```python
from build123d import *

# Parameters (mm, degrees)
EXTRUDE_THIN1_DEPTH = 12.2
SKETCH2_R           = 1.3
CUT_EXTRUDE1_DEPTH  = 28.957288853
SKETCH3_W           = 2
SKETCH3_H           = 10
BOSS_EXTRUDE1_DEPTH = 12.2
FILLET1_R           = 2
SKETCH4_R           = 1.5
CUT_EXTRUDE2_DEPTH  = 32.186695881
SKETCH5_W           = 12.2
SKETCH5_H           = 2
BOSS_EXTRUDE2_DEPTH = 5
SKETCH8_R           = 1.6
CUT_EXTRUDE4_DEPTH  = 3
BOSS_EXTRUDE3_START = 11.4
SKETCH9_W           = 12.2
SKETCH9_H           = 4
SKETCH9_R           = 1.5
BOSS_EXTRUDE3_DEPTH = 11.4
SKETCH10_R          = 1.5
SKETCH10_R_2        = 1.6
CUT_EXTRUDE5_DEPTH  = 12
SKETCH12_R          = 1.9
BOSS_EXTRUDE5_DEPTH = 8
SKETCH13_W          = 1
SKETCH13_H          = 4
CUT_EXTRUDE6_DEPTH  = 37.592485601
FILLET4_R           = 0.5
CUT_EXTRUDE7_REACH  = 38.592
SKETCH14_W          = 4.5
SKETCH14_H          = 1.8
CUT_EXTRUDE8_REACH  = 47.951
SKETCH15_W          = 6
SKETCH15_H          = 8.2


with BuildPart() as part:
    # Sketch1 → Extrude-Thin1 (new body)
    with BuildSketch(Plane(origin=(0, 0, 0), x_dir=(0, 0, -1), z_dir=(1, 0, 0))):
        Polygon((0, 16.6), (0, 11.6), (-18.9, 11.6), (-18.9, -11.6), (0, -11.6), (0, -16.6), (-2, -16.6), (-2, -13.6), (-20.9, -13.6), (-20.9, 13.6), (-2, 13.6), (-2, 16.6), align=None)
    extrude(amount=EXTRUDE_THIN1_DEPTH)

    # Sketch2 → Cut-Extrude1 (cut, through all)
    with BuildSketch(Plane(origin=(0, 0, 18.9), x_dir=(-1, 0, 0), z_dir=(0, 0, -1))):
        with Locations(Location((-6.05, -5.15, 0), (0, 0, 90))):
            Circle(SKETCH2_R)
    extrude(amount=-CUT_EXTRUDE1_DEPTH, mode=Mode.SUBTRACT)

    # Sketch3 → Boss-Extrude1 (add)
    with BuildSketch(Plane(origin=(12.2, 0, 0), x_dir=(0, 0, -1), z_dir=(1, 0, 0))):
        with Locations((-19.9, 16.6)):
            Rectangle(SKETCH3_W, SKETCH3_H)
    extrude(amount=-BOSS_EXTRUDE1_DEPTH)

    # Fillet1
    fillet1_edges = [part.edges().sort_by_distance(p)[0] for p in [
        (6.1, -13.6, 2),
        (6.1, 13.6, 2),
        (6.1, 13.6, 18.9),
    ]]
    fillet(fillet1_edges, radius=FILLET1_R)

    # Sketch4 → Cut-Extrude2 (cut, through all)
    with BuildSketch(Plane(origin=(0, 0, 18.9), x_dir=(-1, 0, 0), z_dir=(0, 0, -1))):
        with Locations((-6.1, 19.6)):
            Circle(SKETCH4_R)
    extrude(amount=-CUT_EXTRUDE2_DEPTH, mode=Mode.SUBTRACT)

    # Sketch5 → Boss-Extrude2 (add)
    with BuildSketch(Plane(origin=(0, 16.6, 0), x_dir=(1, 0, 0), z_dir=(0, 1, 0))):
        with Locations((6.1, -1)):
            Rectangle(SKETCH5_W, SKETCH5_H)
    extrude(amount=BOSS_EXTRUDE2_DEPTH)

    # Sketch8 → Cut-Extrude4 (cut)
    with BuildSketch(Plane.XY.offset(2)):
        with Locations((6.1, 19.6)):
            Circle(SKETCH8_R)
    extrude(amount=-CUT_EXTRUDE4_DEPTH, mode=Mode.SUBTRACT)

    # Sketch9 → Boss-Extrude3 (add)
    with BuildSketch(Plane(origin=(0, 0, 0), x_dir=(-1, 0, 0), z_dir=(0, 0, -1)).offset(BOSS_EXTRUDE3_START)):
        with Locations((-6.1, 19.6)):
            Rectangle(SKETCH9_W, SKETCH9_H)
        with Locations((-6.1, 19.6)):
            Circle(SKETCH9_R, mode=Mode.SUBTRACT)
    extrude(amount=-BOSS_EXTRUDE3_DEPTH)

    # Sketch10 → Cut-Extrude5 (cut)
    with BuildSketch(Plane(origin=(0, 0, 0), x_dir=(-1, 0, 0), z_dir=(0, 0, -1))):
        with Locations(Location((-6.05, -13.9, 0), (0, 0, 90))):
            Circle(SKETCH10_R)
        with Locations(Location((-6.05, 14.1, 0), (0, 0, 90))):
            Circle(SKETCH10_R_2)
    extrude(amount=-CUT_EXTRUDE5_DEPTH, mode=Mode.SUBTRACT)

    # Sketch12 → Boss-Extrude5 (add)
    with BuildSketch(Plane(origin=(0, 0, 18.9), x_dir=(-1, 0, 0), z_dir=(0, 0, -1))):
        with Locations(Location((-6.05, -5.35, 0), (0, 0, 90))):
            Circle(SKETCH12_R)
    extrude(amount=-BOSS_EXTRUDE5_DEPTH)

    # Sketch13 → Cut-Extrude6 (cut, through all)
    with BuildSketch(Plane(origin=(12.2, 0, 0), x_dir=(0, 0, -1), z_dir=(1, 0, 0))):
        with Locations((10.9, 19.6)):
            Rectangle(SKETCH13_W, SKETCH13_H)
    extrude(amount=-CUT_EXTRUDE6_DEPTH, mode=Mode.SUBTRACT)

    # Fillet4
    fillet4_edges = [part.edges().sort_by_distance(p)[0] for p in [
        (6.05, -7.25, 20.9),
    ]]
    fillet(fillet4_edges, radius=FILLET4_R)

    # Cut-Extrude7: up to this face of the body (flat: up to its plane)
    cut_extrude7_end = Plane(part.part.faces().sort_by_distance((6.1, 0, 18.9))[0])
    # Sketch14 → Cut-Extrude7 (cut, up to the picked face)
    with BuildSketch(Plane(origin=(0, 0, 0), x_dir=(-1, 0, 0), z_dir=(0, 0, -1)), mode=Mode.PRIVATE) as cut_extrude7_sk1:
        with Locations((-6.1, -12.5)):
            Rectangle(SKETCH14_W, SKETCH14_H)
    cut_extrude7_tool1 = split(extrude(cut_extrude7_sk1.sketch, amount=-CUT_EXTRUDE7_REACH, mode=Mode.PRIVATE), bisect_by=cut_extrude7_end, keep=Keep.BOTH, mode=Mode.PRIVATE)
    add(cut_extrude7_tool1.solids().sort_by(Axis((6.1, -12.5, 0), (0, 0, 1)))[0], mode=Mode.SUBTRACT)

    # Cut-Extrude8: up to this face of the body (flat: up to its plane)
    cut_extrude8_end = Plane(part.part.faces().sort_by_distance((1.925, -11.6, 9.45))[0])
    # Sketch15 → Cut-Extrude8 (cut, up to the picked face)
    with BuildSketch(Plane.XZ.offset(13.6), mode=Mode.PRIVATE) as cut_extrude8_sk1:
        with Locations((6.1, 14.3)):
            Rectangle(SKETCH15_W, SKETCH15_H)
    cut_extrude8_tool1 = split(extrude(cut_extrude8_sk1.sketch, amount=-CUT_EXTRUDE8_REACH, mode=Mode.PRIVATE), bisect_by=cut_extrude8_end, keep=Keep.BOTH, mode=Mode.PRIVATE)
    add(cut_extrude8_tool1.solids().sort_by(Axis((6.1, -13.6, 14.3), (0, 1, 0)))[0], mode=Mode.SUBTRACT)


solid = part.part
```
Build history of the part. All positions in model axes, mm. A direction names the side the tool comes from. Round coordinates to 2 decimals unless told otherwise and drop trailing zeros. Loops run counter-clockwise (first coordinate to the right, second up) from the corner with the lowest first, then second, coordinate; pieces in that order, holes last.
Item 1: Drill centre lines: line 1 along Y through (x, z) = (6.1, 0.85); line 2 along X through (y, z) = (-13.5, 16); line 3 along Z through (x, y) = (8.5, 17). Where is each one in solid material? Low to high.
Item 2: Which spindle directions (+Z, -Z, +X, -X, +Y, -Y) get a long thin tool onto all of the face, cutting with end or side? Do faces 5 (the face through (6, 11.6, 9)), 6 (the face through (8.35, -13, 5)), 7 (the face through (2.17, 14.2, 2.57)), 8 (the face through (6, 17.6, -5)). Say none if no direction does.
Item 3: Saw through at C-C (z = -6.5). List the corners of the cut face in (x, y).
Item 4: Saw through at D-D (y = -5.35). List the corners of the cut face in (x, z).
Item 5: Saw through at B-B (x = 1.75). List the corners of the cut face in (y, z), then the cut area to 3 significant figures.
Item 6: Pin check, flat tips, straight feed: P1, Ø0.5, axis at y = -12.5, z = 4, coming from the -X side; P2, Ø0.9, axis at x = 6.5, y = 13.5, coming from the -Z side; P3, Ø6, axis at x = 6, y = 9.5, coming from the +Z side; P4, Ø1, axis at x = 10, y = -10, coming from the -Z side. Stop position of each tip, or through.
Item 7: Two-plate mould, pull along Z, no slides. Class faces 1 (the face through (6.2, 17.9, 18.9)), 2 (the face through (6, 16, 0)), 3 (the face through (6, 21.6, -4)), 4 (the face through (6.01, 14.17, 18.3)): released by +Z, released by -Z, zero draft, split by the parting line, or undercut.
Item 8: Saw through at A-A (y = 19.6). List the corners of the cut face in (x, z).
Worked answers:
1. line 1: y = -16.6 to -15.4, 11.6 to 12.5, 15.7 to 18, 21.2 to 21.6
1. line 2: x = 0 to 3.1, 9.1 to 12.2
1. line 3: z = 0 to 2, 18.9 to 20.9
2. face 5: -Z, +X, -X
2. face 6: -Z
2. face 7: +X, -X, +Y
2. face 8: -Z, +X, -X, -Y
3. outline: (0, 17.6) - (12.2, 17.6) - (12.2, 21.6) - (0, 21.6) - close; hole circle Ø3 at (6.1, 19.6)
4. outline: (0, 18.9) - (12.2, 18.9) - (12.2, 20.9) - (8.45, 20.9) arc R0.5 cw to (7.95, 21.4) - (7.95, 26.9) - (4.15, 26.9) - (4.15, 21.4) arc R0.5 cw to (3.65, 20.9) - (0, 20.9) - close
5. outline: (-16.6, 0) - (-11.6, 0) - (-11.6, 18.9) - (11.6, 18.9) - (11.6, 0) - (17.6, 0) - (17.6, -10.4) - (21.6, -10.4) - (21.6, 2) - (15.6, 2) arc R2 cw to (13.6, 4) - (13.6, 16.9) arc R2 cw to (15.6, 18.9) - (21.6, 18.9) - (21.6, 20.9) - (-13.6, 20.9) - (-13.6, 4) arc R2 cw to (-15.6, 2) - (-16.6, 2) - close
5. area: 212 mm2
6. P1: stops at x = 0
6. P2: stops at z = 12
6. P3: stops at z = 20.9
6. P4: stops at z = 18.9
7. face 1: undercut
7. face 2: released by -Z
7. face 3: zero draft
7. face 4: undercut
8. outline: (0, -10.4) - (4.6, -10.4) - (4.6, 0) - (4.5, 0) - (4.5, 2) - (0, 2) - close; (0, 18.9) - (4.6, 18.9) - (4.6, 20.9) - (0, 20.9) - close; (7.6, -10.4) - (12.2, -10.4) - (12.2, 2) - (7.7, 2) - (7.7, 0) - (7.6, 0) - close; (7.6, 18.9) - (12.2, 18.9) - (12.2, 20.9) - (7.6, 20.9) - close
